CAD build for the part. Positions are in the model's coordinates, mm. A direction names the side the tool comes from. Round coordinates to 2 decimals unless told otherwise and drop trailing zeros. Write each loop counter-clockwise with the first axis right and the second up, starting at its lowest first coordinate (ties: lowest second). Pieces come first, ordered by that corner, then holes. Notation, with made-up numbers: (2.25, -18.5) -> (25.25, -18.5) arc R8 ccw to (25.25, -7.5) -> close; hole circle Ø8 at (-23, 43.25). An arc over 180 degrees is marked (long way). Put each result on its own line as item: value. Start each with the question number.
1. Saw through at C-C on z = 1.75. State how many separate pieces and enclosed holes the cut face has, and give its area (3 significant figures).
2. Pull direction Y, two halves, no side cores. Call faces 1 (the flat face through (4, 9.615, 1)), 2 (the flat face through (24.9, 18, 1)), 3 (the flat face through (-21, -13.5, 1)): pulls with the +Y half, pulls with the -Y half, needs draft (parallel to the pull), parting line crosses it, or undercut.
3. 3-axis set-ups, long thin cutter, end or side, ignore diameter. For faces 4 (the flat face through (-19.9, 17, 1)), 5 (the flat face through (12.4, 1, 2)), 6 (the flat face through (2.07, -7.4, 1.48)), 7 (the flat face through (-12.9, 20, 1)): which of +Z, -Z, +X, -X, +Y, -Y reach the whole face in a straight line?
4. Flat gauge pins, fed straight in: P1, Ø0.9, axis at x = -21.5, z = 1.5, coming from the +Y side; P2, Ø2, axis at x = -21.4, y = -2.89, coming from the -Z side; P3, Ø1, axis at y = 8.5, z = 2, coming from the +X side; P4, Ø1, axis at y = -9, z = 2, coming from the -X side. Where does each tip first touch, or does it go through?
5. Saw through at A-A on x = 14.5. List the corners of the cut face in (y, z), and give its area (3 significant figures).
6. Drill centre lines: line 1 (Y direction, x = -21.4, z = 2); line 2 (Y direction, x = 19, z = 1.25); line 3 (X direction, y = -2, z = 2). Where is each one in solid material? Low to high. Write a range as from..to.
7. Saw through at B-B on y = -9.5. List the corners of the cut face in (x, z).
from build123d import *

# Parameters (mm, degrees)
SKETCH_1_R          = 1.8
EXTRUDE_1_DEPTH     = 3
SKETCH_2_W          = 3
SKETCH_2_H          = 27
CUT_EXTRUDE_1_DEPTH = 2
SKETCH_3_W          = 6
SKETCH_3_H          = 3
EXTRUDE_2_DEPTH     = 5
SKETCH_4_W          = 6
SKETCH_4_H          = 3
EXTRUDE_3_DEPTH     = 5
SKETCH_5_W          = 6
SKETCH_5_H          = 3
CUT_EXTRUDE_2_DEPTH = 1
SKETCH_6_W          = 6
SKETCH_6_H          = 3
CUT_EXTRUDE_3_DEPTH = 1
SKETCH_8_W          = 3
SKETCH_8_H          = 19
CUT_EXTRUDE_4_DEPTH = 1.5
EXTRUDE_5_DEPTH     = 3
FILLET_2_R          = 1
CHAMFER_1_SIZE      = 0.5
EXTRUDE_START       = -3
SKETCH_11_R         = 1.8
EXTRUDE_6_DEPTH     = 3
SKETCH_12_R         = 1.4
CUT_EXTRUDE_5_DEPTH = 3


with BuildPart() as part:
    # 草图1 → 凸台-拉伸1 (new body)
    with BuildSketch(Plane.XY):
        Polygon((24.9, -12.5), (15.9, -12.5), (15.9, 14.5), (24.9, 14.5), (24.9, 21.5), (2.1, 21.5), (2.1, 18.7), (-12.9, 18.7), (-12.9, 21.5), (-19.9, 21.5), (-19.9, 11.5), (-22.9, 11.5), (-25.9, 8.5), (-25.9, -10.5), (-22.9, -13.5), (-19.9, -13.5), (-19.9, -26.5), (-9.9, -26.5), (-9.9, -23.7), (4.1, -23.7), (4.1, -26.5), (19.9, -26.5), (19.9, -21.5), (24.9, -21.5), align=None)
        with Locations((-21.4, -1.053344625)):
            Circle(SKETCH_1_R, mode=Mode.SUBTRACT)
        with BuildLine():
            Line((3.499503129, 9.537046136), (-15.209877372, -2.33076439))
            ThreePointArc((-15.209877372, -2.33076439), (-15.380180828, -2.512061787), (-15.442052841, -2.752984736))
            Line((-15.442052841, -2.752984736), (-15.442052841, -4.530228968))
            ThreePointArc((-15.442052841, -4.530228968), (-15.175347113, -4.972466215), (-14.65975771, -4.942914635))
            Line((-14.65975771, -4.942914635), (5.287871242, 8.702140123))
            ThreePointArc((5.287871242, 8.702140123), (5.483249029, 9.262570784), (5.005576111, 9.61482579))
            Line((5.005576111, 9.61482579), (3.767327661, 9.61482579))
            ThreePointArc((3.767327661, 9.61482579), (3.627882641, 9.594987311), (3.499503129, 9.537046136))
        make_face(mode=Mode.SUBTRACT)
        with BuildLine():
            Line((7.966853478, 2.623077919), (-5.180839485, -13.033716755))
            ThreePointArc((-5.180839485, -13.033716755), (-5.267752705, -13.184156416), (-5.297938704, -13.355255232))
            Line((-5.297938704, -13.355255232), (-5.297938704, -14.80023138))
            ThreePointArc((-5.297938704, -14.80023138), (-4.96903752, -15.270045381), (-4.415037923, -15.121769857))
            Line((-4.415037923, -15.121769857), (8.732655041, 0.535024817))
            ThreePointArc((8.732655041, 0.535024817), (8.81956826, 0.685464478), (8.849754259, 0.856563293))
            Line((8.849754259, 0.856563293), (8.849754259, 2.301539442))
            ThreePointArc((8.849754259, 2.301539442), (8.520853075, 2.771353443), (7.966853478, 2.623077919))
        make_face(mode=Mode.SUBTRACT)
    extrude(amount=EXTRUDE_1_DEPTH)

    # 草图2 → 切除-拉伸1 (cut)
    with BuildSketch(Plane(origin=(15.9, 0, 0), x_dir=(0, 0, -1), z_dir=(1, 0, 0))):
        with Locations((-1.5, 1)):
            Rectangle(SKETCH_2_W, SKETCH_2_H)
    extrude(amount=-CUT_EXTRUDE_1_DEPTH, mode=Mode.SUBTRACT)

    # 草图3 → 凸台-拉伸2 (add)
    with BuildSketch(Plane.XZ.offset(-14.5)):
        with Locations((16.9, 1.5)):
            Rectangle(SKETCH_3_W, SKETCH_3_H)
    extrude(amount=EXTRUDE_2_DEPTH)

    # 草图4 → 凸台-拉伸3 (add)
    with BuildSketch(Plane(origin=(0, -12.5, 0), x_dir=(1, 0, 0), z_dir=(0, 1, 0))):
        with Locations((16.9, -1.5)):
            Rectangle(SKETCH_4_W, SKETCH_4_H)
    extrude(amount=EXTRUDE_3_DEPTH)

    # 草图5 → 切除-拉伸2 (cut)
    with BuildSketch(Plane(origin=(0, -7.5, 0), x_dir=(1, 0, 0), z_dir=(0, 1, 0))):
        with Locations((16.9, -1.5)):
            Rectangle(SKETCH_5_W, SKETCH_5_H)
    extrude(amount=-CUT_EXTRUDE_2_DEPTH, mode=Mode.SUBTRACT)

    # 草图6 → 切除-拉伸3 (cut)
    with BuildSketch(Plane.XZ.offset(-9.5)):
        with Locations((16.9, 1.5)):
            Rectangle(SKETCH_6_W, SKETCH_6_H)
    extrude(amount=-CUT_EXTRUDE_3_DEPTH, mode=Mode.SUBTRACT)

    # 草图8 → 切除-拉伸4 (cut)
    with BuildSketch(Plane(origin=(13.9, 0, 0), x_dir=(0, 0, -1), z_dir=(1, 0, 0))):
        with Locations((-1.5, 1)):
            Rectangle(SKETCH_8_W, SKETCH_8_H)
    extrude(amount=-CUT_EXTRUDE_4_DEPTH, mode=Mode.SUBTRACT)

    # 草图10 → 凸台-拉伸5 (add)
    with BuildSketch(Plane.XY.offset(3)):
        Polygon((-25.9, -10.5), (-22.9, -13.5), (-33.008159317, -25.40304294), (-33.008159317, -13.5), (-25.9, 8.5), align=None)
    extrude(amount=-EXTRUDE_5_DEPTH)

    # 圆角2
    fillet_2_edges = [part.edges().sort_by_distance(p)[0] for p in [
        (-33.008159317, -25.40304294, 1.5),
    ]]
    fillet(fillet_2_edges, radius=FILLET_2_R)

    # 倒角1
    chamfer_1_edges = [part.edges().sort_by_distance(p)[0] for p in [
        (24.9, -21.5, 1.5),
        (24.9, 21.5, 1.5),
        (24.9, 14.5, 1.5),
        (24.9, -12.5, 1.5),
    ]]
    chamfer(chamfer_1_edges, length=CHAMFER_1_SIZE)

    # 草图11 → 凸台-拉伸6 (add)
    with BuildSketch(Plane.XY.offset(3).offset(EXTRUDE_START)):
        with Locations((-21.4, -1.053344625)):
            Circle(SKETCH_11_R)
    extrude(amount=EXTRUDE_6_DEPTH)

    # 草图12 → 切除-拉伸5 (cut)
    with BuildSketch(Plane(origin=(175.843153128, -50.872452405, 3), x_dir=(1, 0, 0), z_dir=(0, 0, 1))):
        with Locations((-197.243153128, 47.987065257)):
            Circle(SKETCH_12_R)
    extrude(amount=-CUT_EXTRUDE_5_DEPTH, mode=Mode.SUBTRACT)


solid = part.part
Return value:
1. separate pieces: 1
1. enclosed holes: 3
1. area: 1,950 mm^2
2. face 1: undercut
2. face 2: needs draft
2. face 3: pulls with the -Y half
3. face 4: +Z, -Z, -X, +Y
3. face 5: +Z, -Z, +X
3. face 6: +Z, -Z
3. face 7: +Z, -Z, +Y
4. P1: stops at y = 11.5
4. P2: passes through
4. P3: stops at x = 12.4
4. P4: stops at x = -31.72
5. outline: (-26.5, 0) -> (-8.5, 0) -> (-8.5, 3) -> (-26.5, 3) -> close; (10.5, 0) -> (21.5, 0) -> (21.5, 3) -> (10.5, 3) -> close
5. area: 87.0 mm^2
6. line 1: y = -13.5..-4.29, -1.49..11.5
6. line 2: y = -26.5..-8.5, 10.5..21.5
6. line 3: x = -29.29..-22.48, -20.32..-14.69, -10.36..4.08, 6.6..12.4
7. outline: (-31.72, 0) -> (-2.21, 0) -> (-2.21, 3) -> (-31.72, 3) -> close; (0.31, 0) -> (19.9, 0) -> (19.9, 3) -> (0.31, 3) -> close
